from build123d import *

# Parameters (mm, degrees)
SKETCH1_W                                      = 89.98
SKETCH1_H                                      = 60.99
BASE_FLANGE1_DEPTH                             = 0.5
EDGE_FLANGE1_STRIP_W                           = 3.51892
EDGE_FLANGE1_STRIP_H                           = 0.5
EDGE_FLANGE1_STRIP_CUT_DEPTH                   = 89.98
EDGE_FLANGE1_STRIP_2_W                         = 3.51892
EDGE_FLANGE1_STRIP_2_H                         = 0.5
EDGE_FLANGE1_STRIP_CUT_2_DEPTH                 = 89.98
EDGE_FLANGE1_DEPTH                             = 89.98
EDGE_FLANGE1_BEND_DEPTH                        = 89.98
CSK_FOR_M2_FLAT_HEAD_MACHINE_SCREW1_AT_2_COUNT = 2
CSK_FOR_M2_FLAT_HEAD_MACHINE_SCREW1_AT_2_PITCH = 74.5
CSK_FOR_M2_FLAT_HEAD_MACHINE_SCREW2_AT_2_COUNT = 2
CSK_FOR_M2_FLAT_HEAD_MACHINE_SCREW2_AT_2_PITCH = 74.5
FILLET1_R                                      = 2


# Sheet-metal steps are written as plain solids
with BuildPart() as part:
    # Sketch1 → Base-Flange1 (new body)
    with BuildSketch(Plane(origin=(0, 0, 0), x_dir=(1, 0, 0), z_dir=(0, 1, 0))):
        Rectangle(SKETCH1_W, SKETCH1_H)
    extrude(amount=-BASE_FLANGE1_DEPTH)

    # Edge-Flange1 strip (across the edge) → Edge-Flange1 strip cut (cut)
    with BuildSketch(Plane(origin=(44.99, -0.5, 30.495), x_dir=(0, 0, -1), z_dir=(-1, 0, 0))):
        with Locations((-1, -0.25)):
            Rectangle(EDGE_FLANGE1_STRIP_W, EDGE_FLANGE1_STRIP_H)
    extrude(amount=EDGE_FLANGE1_STRIP_CUT_DEPTH, mode=Mode.SUBTRACT)

    # Edge-Flange1 strip 2 (across the edge) → Edge-Flange1 strip cut 2 (cut)
    with BuildSketch(Plane(origin=(-44.99, -0.5, -30.495), x_dir=(0, 0, 1), z_dir=(1, 0, 0))):
        with Locations((-1, -0.25)):
            Rectangle(EDGE_FLANGE1_STRIP_2_W, EDGE_FLANGE1_STRIP_2_H)
    extrude(amount=EDGE_FLANGE1_STRIP_CUT_2_DEPTH, mode=Mode.SUBTRACT)

    # Edge-Flange1 section (across the edge) → Edge-Flange1 (add)
    with BuildSketch(Plane(origin=(44.99, -0.5, 30.495), x_dir=(0, 0, -1), z_dir=(-1, 0, 0))):
        with BuildLine():
            Line((-0.5, 0.75946), (-0.5, 20.42))
            Line((-0.5, 20.42), (0, 20.42))
            Line((0, 20.42), (0, 0.75946))
            ThreePointArc((0, 0.75946), (0.222440684, 0.222440684), (0.75946, 0))
            Line((0.75946, 0), (0.75946, -0.5))
            ThreePointArc((0.75946, -0.5), (-0.131112707, -0.131112707), (-0.5, 0.75946))
        make_face()
    extrude(amount=EDGE_FLANGE1_DEPTH)

    # Edge-Flange1 section 2 (across the edge) → Edge-Flange1 bend (add)
    with BuildSketch(Plane(origin=(-44.99, -0.5, -30.495), x_dir=(0, 0, 1), z_dir=(1, 0, 0))):
        with BuildLine():
            Line((-0.5, 0.75946), (-0.5, 20.42))
            Line((-0.5, 20.42), (0, 20.42))
            Line((0, 20.42), (0, 0.75946))
            ThreePointArc((0, 0.75946), (0.222440684, 0.222440684), (0.75946, 0))
            Line((0.75946, 0), (0.75946, -0.5))
            ThreePointArc((0.75946, -0.5), (-0.131112707, -0.131112707), (-0.5, 0.75946))
        make_face()
    extrude(amount=EDGE_FLANGE1_BEND_DEPTH)

    # Sketch14 → CSK for M2 Flat Head Machine Screw1 (revolve, cut)
    with BuildSketch(Plane(origin=(-37.25, -16.92, 30.995), x_dir=(0, -1, 0), z_dir=(1, 0, 0))):
        Polygon((0, 0), (0, 0.5), (1.2, 0.5), (1.2, 0.577350269), (2.2, 0), align=None)
    csk_for_m2_flat_head_machine_screw1 = revolve(axis=Axis((-37.25, -16.92, 37.345), (0, 0, -1)), mode=Mode.SUBTRACT)

    # CSK for M2 Flat Head Machine Screw1 at 2: CSK for M2 Flat Head Machine Screw1 ×2
    with Locations(*[(i * CSK_FOR_M2_FLAT_HEAD_MACHINE_SCREW1_AT_2_PITCH, 0, 0) for i in range(1, CSK_FOR_M2_FLAT_HEAD_MACHINE_SCREW1_AT_2_COUNT)]):
        add(csk_for_m2_flat_head_machine_screw1, mode=Mode.SUBTRACT)

    # Sketch20 → CSK for M2 Flat Head Machine Screw2 (revolve, cut)
    with BuildSketch(Plane(origin=(37.25, -16.92, -30.995), x_dir=(0, 1, 0), z_dir=(1, 0, 0))):
        Polygon((0, 0), (0, 0.5), (1.2, 0.5), (1.2, 0.577350269), (2.2, 0), align=None)
    csk_for_m2_flat_head_machine_screw2 = revolve(axis=Axis((37.25, -16.92, -37.345), (0, 0, 1)), mode=Mode.SUBTRACT)

    # CSK for M2 Flat Head Machine Screw2 at 2: CSK for M2 Flat Head Machine Screw2 ×2
    with Locations(*[(-i * CSK_FOR_M2_FLAT_HEAD_MACHINE_SCREW2_AT_2_PITCH, 0, 0) for i in range(1, CSK_FOR_M2_FLAT_HEAD_MACHINE_SCREW2_AT_2_COUNT)]):
        add(csk_for_m2_flat_head_machine_screw2, mode=Mode.SUBTRACT)

    # Fillet1
    fillet1_edges = [part.edges().sort_by_distance(p)[0] for p in [
        (44.99, -20.92, 30.745),
        (-44.99, -20.92, 30.745),
        (-44.99, -20.92, -30.745),
        (44.99, -20.92, -30.745),
    ]]
    fillet(fillet1_edges, radius=FILLET1_R)


solid = part.part
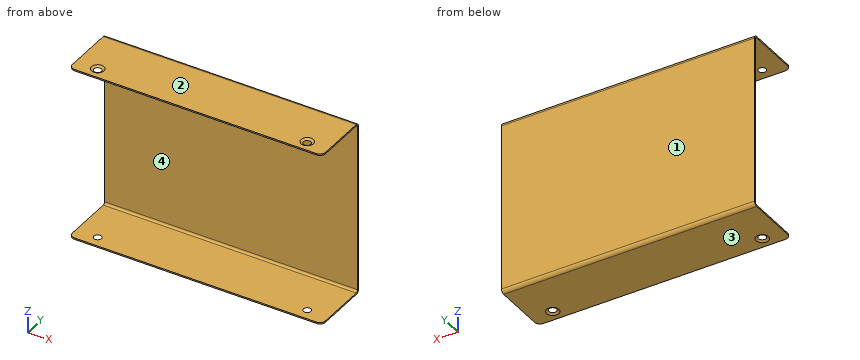
Here's how the part is built. I have some questions about the finished solid (model axes, mm). Face numbers are marked on the shaded views. Coordinates: 2 decimals unless noted, no trailing zeros. Write each loop counter-clockwise with the first axis right and the second up, starting at its lowest first coordinate (ties: lowest second). Pieces come first, ordered by that corner, then holes.
1) If we section it at C-C (x = -37.25): List the corners of the cut face in (y, z) for me (3 decimals), plus the area to 3 significant figures.
Filled in:
outline: (-20.92, -30.995) - (-19.12, -30.995) - (-18.254, -30.495) - (-20.92, -30.495) - close; (-20.92, 30.495) - (-18.254, 30.495) - (-19.12, 30.995) - (-20.92, 30.995) - close; (-15.586, -30.495) - (-14.72, -30.995) - (-1.259, -30.995) arc R1.259 ccw to (0, -29.736) - (0, 29.736) arc R1.259 ccw to (-1.259, 30.995) - (-14.72, 30.995) - (-15.586, 30.495) - (-1.259, 30.495) arc R0.759 cw to (-0.5, 29.736) - (-0.5, -29.736) arc R0.759 cw to (-1.259, -30.495) - close
area: 47.4 mm2
2) I'm going to push flat-ended pins straight in: pin 1 (12 mm diameter, centred on x = 17, z = 15.5, fed in from +Y); pin 2 (8 mm diameter, centred on y = -15, z = -24, fed in from +X); pin 3 (6 mm diameter, centred on x = 22.5, z = 21, fed in from -Y). Where does each tip first touch, or does it pass through?
Filled in:
pin 1: stops at y = 0
pin 2: passes through
pin 3: stops at y = -0.5
3) If we section it at B-B (x = -12.5): List the corners of the cut face in (y, z) for me (3 decimals).
Filled in:
outline: (-20.92, -30.995) - (-1.259, -30.995) arc R1.259 ccw to (0, -29.736) - (0, 29.736) arc R1.259 ccw to (-1.259, 30.995) - (-20.92, 30.995) - (-20.92, 30.495) - (-1.259, 30.495) arc R0.759 cw to (-0.5, 29.736) - (-0.5, -29.736) arc R0.759 cw to (-1.259, -30.495) - (-20.92, -30.495) - close
4) If we section it at D-D (y = -16.92): List the corners of the cut face in (x, z) for me (3 decimals), plus the area to 3 significant figures.
Filled in:
outline: (-44.99, -30.995) - (-39.45, -30.995) - (-38.584, -30.495) - (-44.99, -30.495) - close; (-44.99, 30.495) - (-38.584, 30.495) - (-39.45, 30.995) - (-44.99, 30.995) - close; (-35.916, -30.495) - (-35.05, -30.995) - (35.05, -30.995) - (35.916, -30.495) - close; (-35.916, 30.495) - (35.916, 30.495) - (35.05, 30.995) - (-35.05, 30.995) - close; (38.584, -30.495) - (39.45, -30.995) - (44.99, -30.995) - (44.99, -30.495) - close; (38.584, 30.495) - (44.99, 30.495) - (44.99, 30.995) - (39.45, 30.995) - close
area: 82.9 mm2
5) If I drill on line 1 (Z direction, x = 35, y = -7) (3 decimals); line 2 (Y direction, x = 33, z = -7); line 3 (Z direction, x = -7, y = -0.75), over which ranges is the centre line in solid material (lowest first)?
Filled in:
line 1: z = -30.995 to -30.495, 30.495 to 30.995
line 2: y = -0.5 to 0
line 3: z = -30.89 to -30.3, 30.3 to 30.89
6) Thinking about a two-plate mould opening in Z: for the marked faces 1, 2, 3 and 4, which applies, +Z half, -Z half, draft (parallel to the pull), parting line (faces both ways), or undercut?
Filled in:
face 1: draft
face 2: +Z half
face 3: -Z half
face 4: undercut
7) If we section it at A-A (y = -8.25): List the corners of the cut face in (x, z) for me (3 decimals).
Filled in:
outline: (-44.99, -30.995) - (44.99, -30.995) - (44.99, -30.495) - (-44.99, -30.495) - close; (-44.99, 30.495) - (44.99, 30.495) - (44.99, 30.995) - (-44.99, 30.995) - close
